```python
from build123d import *

# Parameters (mm, degrees)
F0_W      = 1.07834
F0_H      = 1.07834
F1_DEPTH  = 1
F2_W      = 0.7625
F2_H      = 0.7625
F3_DEPTH  = 1.1375
F4_W      = 0.7625
F4_H      = 0.7625
F5_DEPTH  = 1.1375
F6_W      = 0.7625
F6_H      = 0.7625
F7_DEPTH  = 1.1375
F8_W      = 0.7625
F8_H      = 0.7625
F9_DEPTH  = 2.275
F11_DEPTH = 1.07834
F12_W     = 0.7625
F12_H     = 0.7625
F13_DEPTH = 1.1375
F14_W     = 0.7625
F14_H     = 0.7625
F15_DEPTH = 1.1375
F16_W     = 0.7625
F16_H     = 0.7625
F17_DEPTH = 1.1375
F18_W     = 0.7625
F18_H     = 0.7625
F19_DEPTH = 1.1375
F21_DEPTH = 1.07834
F22_W     = 0.7625
F22_H     = 0.7625
F23_DEPTH = 1.1375
F24_W     = 0.7625
F24_H     = 0.7625
F25_DEPTH = 1.1375
F26_W     = 0.7625
F26_H     = 0.7625
F27_DEPTH = 1.1375


with BuildPart() as f1:
    # F0 (on Front) → F1 (new body)
    with BuildSketch(Plane.XZ):
        Rectangle(F0_W, F0_H)
    extrude(amount=F1_DEPTH)

    # F2 (on face) → F3 (join)
    with BuildSketch(Plane(origin=(0, 0, -0.53917), x_dir=(1, 0, 0), z_dir=(0, 0, -1))):
        with Locations((0, 0.38125)):
            Rectangle(F2_W, F2_H)
    extrude(amount=F3_DEPTH)

    # F4 (on face) → F5 (join)
    with BuildSketch(Plane(origin=(-0.53917, 0, 0), x_dir=(0, -1, 0), z_dir=(-1, 0, 0))):
        with Locations((0.38125, 0)):
            Rectangle(F4_W, F4_H)
    extrude(amount=F5_DEPTH)

    # F6 (on face) → F7 (join)
    with BuildSketch(Plane.YZ.offset(0.53917)):
        with Locations((-0.38125, 0)):
            Rectangle(F6_W, F6_H)
    extrude(amount=F7_DEPTH)

    # F8 (on face) → F9 (join)
    with BuildSketch(Plane.XY.offset(0.53917)):
        with Locations((0, -0.38125)):
            Rectangle(F8_W, F8_H)
    extrude(amount=F9_DEPTH)

    # F10 (on face) → F11 (join)
    with BuildSketch(Plane.XY.offset(2.81417)):
        Polygon((0.53917, 0), (0.38125, 0), (-0.53917, 0), (-0.53917, -1), (0.53917, -1), align=None)
    extrude(amount=F11_DEPTH)

    # F12 (on face) → F13 (join)
    with BuildSketch(Plane.YZ.offset(0.53917)):
        with Locations((-0.38125, 3.35334)):
            Rectangle(F12_W, F12_H)
    extrude(amount=F13_DEPTH)

    # F14 (on face) → F15 (join)
    with BuildSketch(Plane.XY.offset(3.89251)):
        with Locations((0, -0.38125)):
            Rectangle(F14_W, F14_H)
    extrude(amount=F15_DEPTH)

    # F16 (on face) → F17 (join)
    with BuildSketch(Plane(origin=(-0.53917, 0, 0), x_dir=(0, -1, 0), z_dir=(-1, 0, 0))):
        with Locations((0.38125, 3.35334)):
            Rectangle(F16_W, F16_H)
    extrude(amount=F17_DEPTH)

    # F18 (on face) → F19 (join)
    with BuildSketch(Plane.YZ.offset(1.67667)):
        with Locations((-0.38125, 0)):
            Rectangle(F18_W, F18_H)
    extrude(amount=F19_DEPTH)

    # F20 (on face) → F21 (join)
    with BuildSketch(Plane.YZ.offset(2.81417)):
        Polygon((0, -0.53917), (0, -0.38125), (0, 0.53917), (-1, 0.53917), (-1, -0.53917), align=None)
    extrude(amount=F21_DEPTH)

    # F22 (on face) → F23 (join)
    with BuildSketch(Plane(origin=(0, 0, -0.53917), x_dir=(1, 0, 0), z_dir=(0, 0, -1))):
        with Locations((3.35334, 0.38125)):
            Rectangle(F22_W, F22_H)
    extrude(amount=F23_DEPTH)

    # F24 (on face) → F25 (join)
    with BuildSketch(Plane.YZ.offset(3.89251)):
        with Locations((-0.38125, 0)):
            Rectangle(F24_W, F24_H)
    extrude(amount=F25_DEPTH)

    # F26 (on face) → F27 (join)
    with BuildSketch(Plane.XY.offset(0.53917)):
        with Locations((3.35334, -0.38125)):
            Rectangle(F26_W, F26_H)
    extrude(amount=F27_DEPTH)


solid = f1.part
```
Can you work these out from the model? Positions are in its coordinate system, mm. Round coordinates to 2 decimals unless told otherwise and drop trailing zeros. Loops run counter-clockwise (first coordinate to the right, second up) from the corner with the lowest first, then second, coordinate; pieces in that order, holes last. Notation, with made-up numbers: M -13,25 L 38,25 A33 cw 38,59 Z; hole C 5,-13.5 d3. An arc over 180 degrees is marked long. Answer as a JSON object with one key per item and string values. Group by question number.
Q1. Imagine slicing it at D-D, the plane z = 2. Please give me the cut outline in (x, y).
Q2. Imagine slicing it at C-C, the plane x = 3.5. Please give me the cut outline in (y, z), then the cut area to 3 significant figures.
Q3. Will these pins go through, and if not, where does the flat tip stop? pin 1 (0.8 mm diameter, centred on x = 4.5, z = 0, fed in from -Y); pin 2 (0.6 mm diameter, centred on y = -0.5, z = 1, fed in from -X).
Q4. Imagine slicing it at B-B, the plane x = 1. Please give me the cut outline in (y, z), then the cut area to 3 significant figures.
Q5. Imagine slicing it at A-A, the plane z = -0.75. Please give me the cut outline in (x, y), then the cut area to 3 significant figures.
Q6. Please list where these lines run through material, in increasing order: L1, parallel to X at y = -0.7, z = -1; L2, parallel to X at y = -0.15, z = 0.5.
Findings:
{
 "1": {"outline": "M -0.38,-0.76 L 0.38,-0.76 L 0.38,0 L -0.38,0 Z"},
 "2": {"outline": "M -1,-0.54 L -0.76,-0.54 L -0.76,-1.68 L 0,-1.68 L 0,1.68 L -0.76,1.68 L -0.76,0.54 L -1,0.54 Z", "area": "2.81 mm2"},
 "3": {"pin 1": "stops at y = -0.76", "pin 2": "stops at x = -0.38"},
 "4": {"outline": "M -0.76,-0.38 L 0,-0.38 L 0,0.38 L -0.76,0.38 Z; M -0.76,2.97 L 0,2.97 L 0,3.73 L -0.76,3.73 Z", "area": "1.16 mm2"},
 "5": {"outline": "M -0.38,-0.76 L 0.38,-0.76 L 0.38,0 L -0.38,0 Z; M 2.97,-0.76 L 3.73,-0.76 L 3.73,0 L 2.97,0 Z", "area": "1.16 mm2"},
 "6": {"L1": "x = -0.38 to 0.38, 2.97 to 3.73", "L2": "x = -0.54 to 0.54, 2.81 to 3.89"}
}
